```python
from build123d import *

# Parameters (mm, degrees)
F1_DEPTH = 25
F2_R     = 2
F3_R     = 1
F4_DEPTH = 8


with BuildPart() as f1:
    # F0 (on Top) → F1 (new body)
    with BuildSketch(Plane.XY):
        with BuildLine():
            ThreePointArc((10, 2.5), (8.535534, 6.035534), (5, 7.5))
            Line((5, 7.5), (-5, 7.5))
            ThreePointArc((-5, 7.5), (-8.535534, 6.035534), (-10, 2.5))
            Line((-10, 2.5), (-10, -2.5))
            ThreePointArc((-10, -2.5), (-8.535534, -6.035534), (-5, -7.5))
            Line((-5, -7.5), (5, -7.5))
            ThreePointArc((5, -7.5), (8.535534, -6.035534), (10, -2.5))
            Line((10, -2.5), (10, 2.5))
        make_face()
    extrude(amount=F1_DEPTH)

    # F2
    f2_edges = [f1.edges().sort_by_distance(p)[0] for p in [
        (0, 7.5, 25),
        (0, 7.5, 0),
    ]]
    fillet(f2_edges, radius=F2_R)

    # F3 (on face) → F4 (join)
    with BuildSketch(Plane.XY.offset(25)):
        Circle(F3_R)
    extrude(amount=F4_DEPTH)


solid = f1.part
```
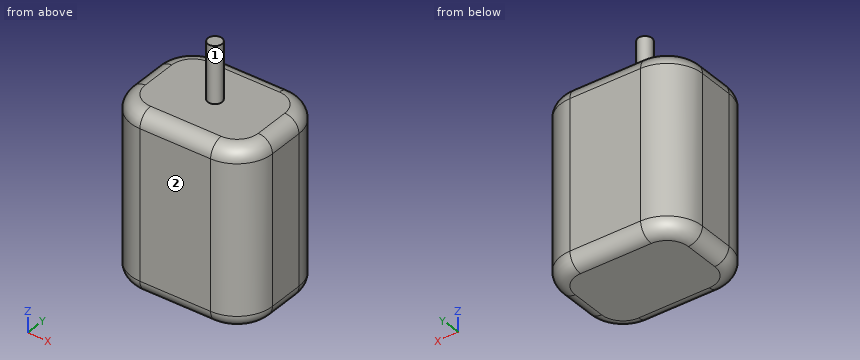
The listing builds one solid part. Answer for the finished solid, in the listing's coordinates (mm). Face numbers are marked on the shaded views. A direction names the side the tool comes from. Coordinates: 2 decimals unless noted, no trailing zeros. Loops run counter-clockwise (first coordinate to the right, second up) from the corner with the lowest first, then second, coordinate; pieces in that order, holes last. Notation, with made-up numbers: M -9,8.25 L 5,8.25 A27 cw 5,42.25 Z; hole C 86.5,16 d11. An arc over 180 degrees is marked long. Answer as a JSON object with one key per item and string values. Group by question number.
Item 1: Section C-C (y = 0) is taken. Write down the section's boundary in (x, z), and give its area (3 significant figures).
Item 2: Section D-D (x = 2.75) is taken. Write down the section's boundary in (y, z), and give its area (3 significant figures).
Item 3: Section B-B (z = 15) is taken. Write down the section's boundary in (x, y).
Item 4: Consider L1, parallel to Z at x = -3, y = -1.5; L2, parallel to Y at x = -5.25, z = 11.5; L3, parallel to Z at x = 9, y = -2. Determine where each line is inside the solid, lowest interval first.
Item 5: Section A-A (x = 0) is taken. Write down the section's boundary in (y, z).
Item 6: Which of the six approach directions +Z, -Z, +X, -X, +Y, -Y give full straight-line access (tool end or side, diameter ignored) to the marked faces 1 and 2?
Solved:
{
 "1": {"outline": "M -10,2 A2 ccw -8,0 L 8,0 A2 ccw 10,2 L 10,23 A2 ccw 8,25 L 1,25 L 1,33 L -1,33 L -1,25 L -8,25 A2 ccw -10,23 Z", "area": "513 mm2"},
 "2": {"outline": "M -7.5,2 A2 ccw -5.5,0 L 5.5,0 A2 ccw 7.5,2 L 7.5,23 A2 ccw 5.5,25 L -5.5,25 A2 ccw -7.5,23 Z", "area": "372 mm2"},
 "3": {"outline": "M -10,-2.5 A5 ccw -5,-7.5 L 5,-7.5 A5 ccw 10,-2.5 L 10,2.5 A5 ccw 5,7.5 L -5,7.5 A5 ccw -10,2.5 Z"},
 "4": {"L1": "z = 0 to 25", "L2": "y = -7.49 to 7.49", "L3": "z = 0.27 to 24.73"},
 "5": {"outline": "M -7.5,2 A2 ccw -5.5,0 L 5.5,0 A2 ccw 7.5,2 L 7.5,23 A2 ccw 5.5,25 L 1,25 L 1,33 L -1,33 L -1,25 L -5.5,25 A2 ccw -7.5,23 Z"},
 "6": {"face 1": "+Z", "face 2": "+Z, -Z, +X, -X, -Y"}
}
